```python
from build123d import *

# Parameters (mm, degrees)
F0_R      = 4
F1_DEPTH  = 8
F2_W      = 10
F2_H      = 33.13
F3_DEPTH  = 3
F4_R      = 1.5
F5_DEPTH  = 26
F6_W      = 20.15
F6_H      = 28.71
F7_DEPTH  = 9
F8_R      = 11
F9_DEPTH  = 11
F10_R     = 1.25
F11_DEPTH = 47.351
F12_R     = 11
F13_DEPTH = 11


# Not quite as in the source:
# - a pattern or mirror of a feature is missing from the dataset's text; its kind, count and spacing are read off the source's solid


with BuildPart() as f1:
    # F0 (on Top) → F1 (new body)
    with BuildSketch(Plane.XY):
        Polygon((55.25, -26.455), (55.25, 26.455), (45.74, 26.455), (45.74, 18.175), (19.25, 18.175), (19.25, 26.455), (-24.73, 26.455), (-24.73, 14.955), (-55.25, 14.955), (-55.25, -18.175), (-24.75, -18.175), (-24.75, -26.455), (19.25, -26.455), (19.25, -18.175), (45.74, -18.175), (45.74, -26.455), align=None)
        with Locations((49.26, -13)):
            Circle(F0_R, mode=Mode.SUBTRACT)
        with Locations((-50.74, 0)):
            Circle(F0_R, mode=Mode.SUBTRACT)
        with Locations((49.26, 13)):
            Circle(F0_R, mode=Mode.SUBTRACT)
    extrude(amount=F1_DEPTH)

    # F2 (on face) → F3 (join)
    with BuildSketch(Plane.XY.offset(8)):
        with Locations((-40.25, -1.61)):
            Rectangle(F2_W, F2_H)
    extrude(amount=F3_DEPTH)

    # F4 (on Front) → F5 (join, symmetric)
    with BuildSketch(Plane.XZ):
        with Locations((-38.47, 7.2)):
            Circle(F4_R)
    extrude(amount=F5_DEPTH, both=True)

    # F6 (on face) → F7 (join)
    with BuildSketch(Plane.XY.offset(8)):
        with Locations((-26.825, -0.5)):
            Rectangle(F6_W, F6_H)
    extrude(amount=F7_DEPTH)

    # F8 (on face) → F9 (join)
    with BuildSketch(Plane.XZ.offset(18.175)):
        with Locations((-38.47, 7.2)):
            Circle(F8_R)
    f9 = extrude(amount=F9_DEPTH)

    # F9_copies: F9 across plane
    add(f9.mirror(Plane.ZX))

    # F10 (on face) → F11 (cut, through all)
    with BuildSketch(Plane.XZ.offset(18.175)):
        with Locations((32.76, 6.375)):
            Circle(F10_R)
    extrude(amount=-F11_DEPTH, mode=Mode.SUBTRACT)

    # F12 (on face) → F13 (join)
    with BuildSketch(Plane.XZ.offset(18.175)):
        with Locations((32.76, 6.375)):
            Circle(F12_R)
    f13 = extrude(amount=F13_DEPTH)

    # F13_copies: F13 across plane
    add(f13.mirror(Plane.ZX))


solid = f1.part
```
Read the model definition and answer for the solid it produces. Units are mm, in the model's axes. A direction names the side the tool comes from. Coordinates: 2 decimals unless noted, no trailing zeros. Order: outer loops, then holes, each group sorted by start corner. A loop starts at its lowest first (then second) coordinate and runs counter-clockwise, first axis right, second up. Notation, with made-up numbers: (62, 18.25) - (89, 18.25) arc R29 cw to (89, 56.25) - close; hole circle Ø1 at (2, 39). An arc over 180 degrees is marked (long way). Answer as a JSON object with one key per item and string values. Group by question number.
Item 1: The mould has two halves that part along Y. Classify faces 1 (the face through (-39, -29.175, 7)), 2 (the face through (33, -18.175, -2)), 3 (the face through (-24.75, -22, 4)): +Y half, -Y half, draft (parallel to the pull), parting line (faces both ways), or undercut.
Item 2: A tool of negligible diameter and unlimited length cuts with its end or side. For faces 4 (the face through (30.375, 23.598, -4.363)), 5 (the face through (-35.25, -17, 9)), 6 (the face through (-3, -26.455, 4)), from which of +Z, -Z, +X, -X, +Y, -Y can it reach the whole face along a straight path? Write none if from no direction.
Item 3: Consider probe 1 along Y at (x, z) = (49.26, 2.5) (3 decimals); probe 2 along X at (y, z) = (19, 3.25); probe 3 along Y at (x, z) = (-50.74, 6) (3 decimals). Determine where each line is inside the solid, lowest interval first. Write a range as from..to.
Item 4: Section C-C (x = 49.26) is taken. Give the vertices of the cut face in (y, z) (3 decimals), plus the area to 3 significant figures.
Item 5: Section A-A (x = 32.76) is taken. Give the vertices of the cut face in (y, z) (3 decimals), plus the area to 3 significant figures.
Item 6: Section B-B (y = 0) is taken. Give the vertices of the cut face in (x, z) (3 decimals).
Item 7: Flat-ended cylindrical pins translate along their axes: P1, Ø4, axis at x = 17, z = -1, coming from the -Y side (3 decimals); P2, Ø1.5, axis at x = -15, y = 11.5, coming from the +Z side; P3, Ø11, axis at x = -41.5, y = -2.5, coming from the +Z side; P4, Ø7, axis at x = 49.26, y = 13, coming from the -Z side. Find the tip coordinate at first contact, or state that the pin passes through.
Item 8: Section D-D (z = 14.25) is taken. Give the vertices of the cut face in (x, y) (3 decimals).
Results are:
{
 "1": {"face 1": "-Y half", "face 2": "undercut", "face 3": "draft"},
 "2": {"face 4": "+Y", "face 5": "+Z, +X", "face 6": "+Z, -Z, -Y"},
 "3": {"probe 1": "y = -26.455..-17, -9..9, 17..26.455", "probe 2": "x = -48.74..-28.2, -24.73..19.25, 22.21..43.31, 45.74..55.25", "probe 3": "y = -18.175..-4, 4..14.955"},
 "4": {"outline": "(-26.455, 0) - (-17, 0) - (-17, 8) - (-26.455, 8) - close; (-9, 0) - (9, 0) - (9, 8) - (-9, 8) - close; (17, 0) - (26.455, 0) - (26.455, 8) - (17, 8) - close", "area": "295 mm^2"},
 "5": {"outline": "(-29.175, -4.625) - (-18.175, -4.625) - (-18.175, 0) - (18.175, 0) - (18.175, -4.625) - (29.175, -4.625) - (29.175, 17.375) - (18.175, 17.375) - (18.175, 8) - (-18.175, 8) - (-18.175, 17.375) - (-29.175, 17.375) - close; hole (-18.175, 5.125) - (18.175, 5.125) - (18.175, 7.625) - (-18.175, 7.625) - close", "area": "684 mm^2"},
 "6": {"outline": "(-55.25, 0) - (-54.74, 0) - (-54.74, 8) - (-55.25, 8) - close; (-46.74, 0) - (55.25, 0) - (55.25, 8) - (-16.75, 8) - (-16.75, 17) - (-36.9, 17) - (-36.9, 11) - (-45.25, 11) - (-45.25, 8) - (-46.74, 8) - close; hole circle Ø2.5 at (32.76, 6.375)"},
 "7": {"P1": "stops at y = -26.455", "P2": "stops at z = 8", "P3": "stops at z = 17", "P4": "passes through"},
 "8": {"outline": "(-46.914, -29.175) - (-30.026, -29.175) - (-30.026, -18.175) - (-46.914, -18.175) - close; (-46.914, 18.175) - (-30.026, 18.175) - (-30.026, 29.175) - (-46.914, 29.175) - close; (-36.9, -14.855) - (-16.75, -14.855) - (-16.75, 13.855) - (-36.9, 13.855) - close; (25.08, -29.175) - (40.44, -29.175) - (40.44, -18.175) - (25.08, -18.175) - close; (25.08, 18.175) - (40.44, 18.175) - (40.44, 29.175) - (25.08, 29.175) - close"}
}
